from build123d import *

# Parameters (mm, degrees)
SKETCH1_R                                       = 5
SKETCH1_R_2                                     = 2.5
BOSS_EXTRUDE2_DEPTH                             = 12
SKETCH3_R                                       = 11
SKETCH3_R_2                                     = 5
BOSS_EXTRUDE3_DEPTH                             = 2
FILLET1_R                                       = 0.5
CUT_EXTRUDE1_DEPTH                              = 2
CIRPATTERN1_COUNT                               = 4
CSK_FOR_M3_FLAT_HEAD_MACHINE_SCREW2_D           = 3.2
CSK_FOR_M3_FLAT_HEAD_MACHINE_SCREW2_CSINK_D     = 5
CSK_FOR_M3_FLAT_HEAD_MACHINE_SCREW2_CSINK_ANGLE = 120


with BuildPart() as part:
    # Sketch1 → Boss-Extrude2 (new body)
    with BuildSketch(Plane.XY):
        Circle(SKETCH1_R)
        Circle(SKETCH1_R_2, mode=Mode.SUBTRACT)
    extrude(amount=BOSS_EXTRUDE2_DEPTH)

    # Sketch3 → Boss-Extrude3 (add)
    with BuildSketch(Plane.XY):
        Circle(SKETCH3_R)
        Circle(SKETCH3_R_2, mode=Mode.SUBTRACT)
    extrude(amount=BOSS_EXTRUDE3_DEPTH)

    # Fillet1
    fillet1_edges = [part.edges().sort_by_distance(p)[0] for p in [
        (-5, 0, 2),
    ]]
    fillet(fillet1_edges, radius=FILLET1_R)

    # Sketch5 → Cut-Extrude1 (cut)
    with BuildSketch(Plane.XY.offset(2)):
        with BuildLine():
            ThreePointArc((-1.419675746, 8.126931818), (-0.963133646, 7.199762608), (0, 6.825))
            Line((0, 6.825), (0, 8.25))
            ThreePointArc((0, 8.25), (-0.7125, 8.219175369), (-1.419675746, 8.126931818))
        make_face()
        with BuildLine():
            Line((0, 8.25), (0, 6.825))
            ThreePointArc((0, 6.825), (0.963133646, 7.199762608), (1.419675746, 8.126931818))
            ThreePointArc((1.419675746, 8.126931818), (0.7125, 8.219175369), (0, 8.25))
        make_face()
        with BuildLine():
            ThreePointArc((-1.419675746, 8.126931818), (-0.7125, 8.219175369), (0, 8.25))
            Line((0, 8.25), (0, 9.675))
            ThreePointArc((0, 9.675), (-1.050237392, 9.213133646), (-1.419675746, 8.126931818))
        make_face()
        with BuildLine():
            Line((0, 9.675), (0, 8.25))
            ThreePointArc((0, 8.25), (0.7125, 8.219175369), (1.419675746, 8.126931818))
            ThreePointArc((1.419675746, 8.126931818), (1.423668314, 8.188408351), (1.425, 8.25))
            ThreePointArc((1.425, 8.25), (1.007627163, 9.257627163), (0, 9.675))
        make_face()
    cut_extrude1 = extrude(amount=-CUT_EXTRUDE1_DEPTH, mode=Mode.SUBTRACT)

    # CirPattern1: Cut-Extrude1 ×4 about axis
    cirpattern1_axis = Axis((0, 0, 0), (0, 0, 1))
    for i in range(1, CIRPATTERN1_COUNT):
        add(cut_extrude1.rotate(cirpattern1_axis, i * 360 / CIRPATTERN1_COUNT), mode=Mode.SUBTRACT)

    # CSK for M3 Flat Head Machine Screw2 (through all)
    with Locations(Plane(origin=(4.999975674, -0.015596745, 7.232142879), x_dir=(0.003119349, 0.999995135, 0), z_dir=(0.999995135, -0.003119349, 0))):
        with Locations((0, 0)):
            CounterSinkHole(CSK_FOR_M3_FLAT_HEAD_MACHINE_SCREW2_D / 2, CSK_FOR_M3_FLAT_HEAD_MACHINE_SCREW2_CSINK_D / 2, counter_sink_angle=CSK_FOR_M3_FLAT_HEAD_MACHINE_SCREW2_CSINK_ANGLE)


solid = part.part
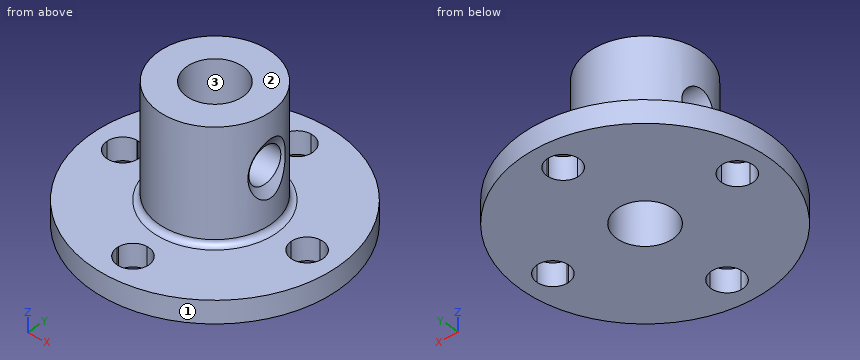
The listing builds one solid part. Answer for the finished solid, in the listing's coordinates (mm). Face numbers are marked on the shaded views. Give positions to 0.01 mm unless a question says otherwise; leave off trailing zeros. Write each loop counter-clockwise with the first axis right and the second up, starting at its lowest first coordinate (ties: lowest second). Pieces come first, ordered by that corner, then holes. Notation, with made-up numbers: (64.25, -4) - (78.25, -4) arc R21 ccw to (78.25, 32) - close; hole circle Ø4 at (82.25, 16). An arc over 180 degrees is marked (long way). Use a Markdown table: item, result.
1. For a pull along X with two mould halves and no side action, classify the marked faces 1, 2 and 3 as released by +X, released by -X, zero draft, split by the parting line, or undercut.
Values follow:
| item | result |
|---|---|
| face 1 | split by the parting line |
| face 2 | zero draft |
| face 3 | undercut |
2. Section A-A on z = 10.5 is taken. Write down the section's boundary in (x, y).
Values follow:
| item | result |
|---|---|
| outline | circle Ø10 at (0, 0); hole circle Ø5 at (0, 0) |
3. Find the intervals of material crossed by probe 1 along Y at (x, z) = (0, 7.5); probe 2 along Z at (x, y) = (-4.25, -4.5), in increasing order. Write a range as from..to.
Values follow:
| item | result |
|---|---|
| probe 1 | y = -5..-2.5, 2.5..5 |
| probe 2 | z = 0..2 |
4. Each of these flat-tipped pins is pushed along its axis until it touches: P1, Ø1.5, axis at y = 1, z = 1.5, coming from the -X side; P2, Ø2, axis at x = 3, z = 5, coming from the -Y side; P3, Ø8, axis at x = 0, y = 0, coming from the -Z side; P4, Ø2, axis at y = -7.5, z = 2.5, coming from the +X side. Where does it stop, or does it pass through?
Values follow:
| item | result |
|---|---|
| P1 | stops at x = -11 |
| P2 | stops at y = -4.58 |
| P3 | stops at z = 0 |
| P4 | stops at x = 8.77 |
